Read the model definition and answer for the solid it produces. Units are mm, in the model's axes. A direction names the side the tool comes from. Coordinates: 2 decimals unless noted, no trailing zeros. Write each loop counter-clockwise with the first axis right and the second up, starting at its lowest first coordinate (ties: lowest second). Pieces come first, ordered by that corner, then holes. Notation, with made-up numbers: (86, 53) - (144, 53) arc R8 ccw to (144, 68) - close; hole circle Ø3 at (57.5, 17). An arc over 180 degrees is marked (long way). Return JSON: item names as keys, results as strings.
```python
from build123d import *

# Parameters (mm, degrees)
F0_W     = 152.4
F0_H     = 25.4
F0_R     = 2.6
F0_R_2   = 2.5527
F0_R_3   = 4.7625
F1_DEPTH = 7
F3_DEPTH = 0.2
F4_W     = 1.160611
F4_H     = 18.825986
F5_DEPTH = 0.5
F6_W     = 4
F6_H     = 27.813
F7_DEPTH = 19.812
F8_R     = 1.7891
F9_DEPTH = 4


with BuildPart() as f1:
    # F0 (on Front) → F1 (new body)
    with BuildSketch(Plane.XZ):
        with Locations((0, -12.7)):
            Rectangle(F0_W, F0_H)
        with Locations((-66.675, -12.7)):
            Circle(F0_R, mode=Mode.SUBTRACT)
        with Locations((-21.7079, -5)):
            Circle(F0_R_2, mode=Mode.SUBTRACT)
        with Locations((66.675, -12.7)):
            Circle(F0_R, mode=Mode.SUBTRACT)
        with Locations((3.6921, -5)):
            Circle(F0_R_2, mode=Mode.SUBTRACT)
        with Locations((0, 12.7)):
            Rectangle(F0_W, F0_H)
        with Locations((-66.675, 12.7)):
            Circle(F0_R, mode=Mode.SUBTRACT)
        with Locations((-53.975, 15.875)):
            Circle(F0_R_3, mode=Mode.SUBTRACT)
        with Locations((66.675, 12.7)):
            Circle(F0_R, mode=Mode.SUBTRACT)
        with Locations((53.975, 15.875)):
            Circle(F0_R_3, mode=Mode.SUBTRACT)
    extrude(amount=F1_DEPTH)

    # F0 (on Front) → F3 (cut)
    with BuildSketch(Plane.XZ):
        with Locations((0, -12.7)):
            Rectangle(F0_W, F0_H)
        with Locations((-66.675, -12.7)):
            Circle(F0_R, mode=Mode.SUBTRACT)
        with Locations((-21.7079, -5)):
            Circle(F0_R_2, mode=Mode.SUBTRACT)
        with Locations((66.675, -12.7)):
            Circle(F0_R, mode=Mode.SUBTRACT)
        with Locations((3.6921, -5)):
            Circle(F0_R_2, mode=Mode.SUBTRACT)
        with Locations((0, 12.7)):
            Rectangle(F0_W, F0_H)
        with Locations((-66.675, 12.7)):
            Circle(F0_R, mode=Mode.SUBTRACT)
        with Locations((-53.975, 15.875)):
            Circle(F0_R_3, mode=Mode.SUBTRACT)
        with Locations((66.675, 12.7)):
            Circle(F0_R, mode=Mode.SUBTRACT)
        with Locations((53.975, 15.875)):
            Circle(F0_R_3, mode=Mode.SUBTRACT)
    extrude(amount=-F3_DEPTH, mode=Mode.SUBTRACT)

    # F4 (on face) → F5 (cut)
    with BuildSketch(Plane.XZ.offset(7)):
        with Locations((11.550757, -4.44987)):
            Rectangle(F4_W, F4_H)
    extrude(amount=-F5_DEPTH, mode=Mode.SUBTRACT)

    # F6 (on face) → F7 (join)
    with BuildSketch(Plane(origin=(0, 0, 0), x_dir=(-1, 0, 0), z_dir=(0, 1, 0))):
        with Locations((-44.681652, 8.0931)):
            Rectangle(F6_W, F6_H)
    extrude(amount=F7_DEPTH)

    # F8 (on face) → F9 (cut, through all)
    with BuildSketch(Plane(origin=(42.681652, 0, 0), x_dir=(0, -1, 0), z_dir=(-1, 0, 0))):
        with Locations((-16.8545, -2.8559)):
            Circle(F8_R)
        with Locations((-6.928358, 19.0421)):
            Circle(F8_R)
    extrude(amount=-F9_DEPTH, mode=Mode.SUBTRACT)


solid = f1.part
```
(1) A cutting plane is placed at A-A (z = 12.7). Determine the outline of the cut face in (x, y) (3 decimals).
Answer:
{"outline": "(-76.2, -7) - (-69.275, -7) - (-69.275, 0) - (-76.2, 0) - close; (-64.075, -7) - (-57.525, -7) - (-57.525, 0) - (-64.075, 0) - close; (-50.425, -7) - (50.425, -7) - (50.425, 0) - (46.682, 0) - (46.682, 19.812) - (42.682, 19.812) - (42.682, 0) - (-50.425, 0) - close; (57.525, -7) - (64.075, -7) - (64.075, 0) - (57.525, 0) - close; (69.275, -7) - (76.2, -7) - (76.2, 0) - (69.275, 0) - close"}
(2) A cutting plane is placed at C-C (x = -54.5). Determine the outline of the cut face in (y, z).
Answer:
{"outline": "(-7, -25.4) - (0, -25.4) - (0, 11.14) - (-7, 11.14) - close; (-7, 20.61) - (0, 20.61) - (0, 25.4) - (-7, 25.4) - close"}
(3) Straight lines are drawn through the part: line 1 (Y direction, x = 18, z = 22); line 2 (X direction, y = 13.25, z = 6); line 3 (Z direction, x = 45, y = 14). For each, find the intervals that lie inside material, in ascending order. Write a range as from..to.
Answer:
{"line 1": "-7..0", "line 2": "42.68..46.68", "line 3": "-5.81..22"}
(4) Determine the mould class of faces 6 (the face through (44.654, 15.148, -2.319)), 7 (the face through (-1, -7, 0)), 8 (the face through (69.155, -3.451, 13.481)) for opening direction Y: +Y half, -Y half, draft (parallel to the pull), parting line (faces both ways), or undercut.
Answer:
{"face 6": "undercut", "face 7": "-Y half", "face 8": "draft"}
(5) A cutting plane is placed at D-D (y = -3.75). State how many separate pieces and enclosed holes the cut face has, and give its area (3 significant figures).
Answer:
{"separate pieces": "1", "enclosed holes": "8", "area": "7,470 mm²"}
(6) A cutting plane is placed at B-B (x = 65.5). Determine the outline of the cut face in (y, z).
Answer:
{"outline": "(-7, -25.4) - (0, -25.4) - (0, -15.02) - (-7, -15.02) - close; (-7, -10.38) - (0, -10.38) - (0, 10.38) - (-7, 10.38) - close; (-7, 15.02) - (0, 15.02) - (0, 25.4) - (-7, 25.4) - close"}
(7) Which of the six approach directions +Z, -Z, +X, -X, +Y, -Y give full straight-line access (tool end or side, diameter ignored) to faces 1 (the face through (-1, -3, -25.4)), 2 (the face through (-64.2, -3.5, 13.5)), 3 (the face through (45, 10, -5.813)), 4 (the face through (46.682, 10, 8)), 5 (the face through (42.682, 10, 8))?
Answer:
{"face 1": "-Z, +X, -X, +Y, -Y", "face 2": "+Y, -Y", "face 3": "-Z, +X, -X, +Y", "face 4": "+Z, -Z, +X, +Y", "face 5": "+Z, -Z, -X, +Y"}
(8) Flat-ended cylindrical pins translate along their axes: P1, Ø7, axis at x = 66.675, z = -12.7, coming from the -Y side; P2, Ø10, axis at x = 22.5, z = -18, coming from the +Y side; P3, Ø2, axis at x = 45.5, y = 12, coming from the -Z side; P4, Ø5.5, axis at y = 6.93, z = 19.04, coming from the +X side. Find the tip coordinate at first contact, or state that the pin passes through.
Answer:
{"P1": "y = -7", "P2": "y = 0", "P3": "z = -5.81", "P4": "x = 46.68"}
